Verification items for the finished model (mm, model axes). Coordinates: 2 decimals unless noted, no trailing zeros. Write each loop counter-clockwise with the first axis right and the second up, starting at its lowest first coordinate (ties: lowest second). Pieces come first, ordered by that corner, then holes. Notation, with made-up numbers: (-31.5, 25) -> (-18.5, 25) arc R37 cw to (-18.5, 62) -> close; hole circle Ø3 at (41.25, -6.5). An arc over 180 degrees is marked (long way). Answer in a Markdown table with one row per item.
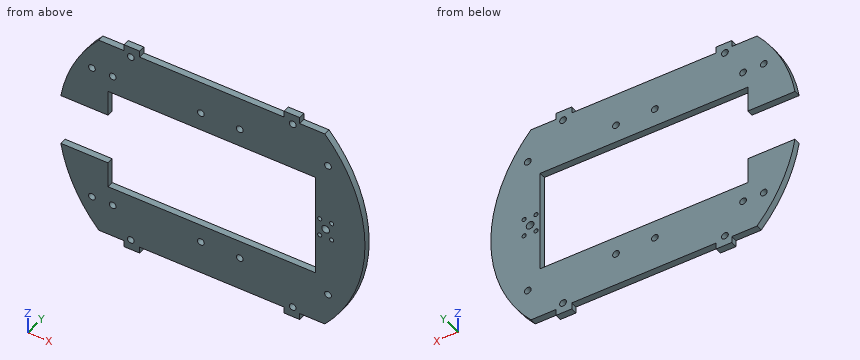
```python
from build123d import *

# Parameters (mm, degrees)
SKETCH1_R           = 1.651
SKETCH1_R_2         = 1.905
SKETCH1_R_3         = 1.016
SKETCH1_W           = 101.6
SKETCH1_H           = 50.8
BOSS_EXTRUDE1_DEPTH = 3.175
SKETCH3_W           = 23.116912814
SKETCH3_H           = 25.4
CUT_EXTRUDE2_DEPTH  = 3.175


with BuildPart() as part:
    # Sketch1 → Boss-Extrude1 (new body)
    with BuildSketch(Plane(origin=(0, 0, 0), x_dir=(1, 0, 0), z_dir=(0, 1, 0))):
        with BuildLine():
            Line((-73.916912814, 12.7), (-73.916912814, -12.7))
            ThreePointArc((-73.916912814, -12.7), (-67.357563081, -32.984218889), (-55.35602635, -50.603461806))
            Line((-55.35602635, -50.603461806), (-42.984152136, -50.603461806))
            Line((-42.984152136, -50.603461806), (-42.984152136, -53.778461806))
            Line((-42.984152136, -53.778461806), (-35.364152136, -53.778461806))
            Line((-35.364152136, -53.778461806), (-35.364152136, -50.603461806))
            Line((-35.364152136, -50.603461806), (35.364152136, -50.603461806))
            Line((35.364152136, -50.603461806), (35.364152136, -53.778461806))
            Line((35.364152136, -53.778461806), (42.984152136, -53.778461806))
            Line((42.984152136, -53.778461806), (42.984152136, -50.603461806))
            Line((42.984152136, -50.603461806), (55.35602635, -50.603461806))
            ThreePointArc((55.35602635, -50.603461806), (75, 0), (55.35602635, 50.603461806))
            Line((55.35602635, 50.603461806), (42.984152136, 50.603461806))
            Line((42.984152136, 50.603461806), (42.984152136, 53.778461806))
            Line((42.984152136, 53.778461806), (35.364152136, 53.778461806))
            Line((35.364152136, 53.778461806), (35.364152136, 50.603461806))
            Line((35.364152136, 50.603461806), (-35.364152136, 50.603461806))
            Line((-35.364152136, 50.603461806), (-35.364152136, 53.778461806))
            Line((-35.364152136, 53.778461806), (-42.984152136, 53.778461806))
            Line((-42.984152136, 53.778461806), (-42.984152136, 50.603461806))
            Line((-42.984152136, 50.603461806), (-55.35602635, 50.603461806))
            ThreePointArc((-55.35602635, 50.603461806), (-67.357563081, 32.984218889), (-73.916912814, 12.7))
        make_face()
        with Locations(Location((13.713087186, 34.29, 0), (0, 0, 270))):
            Circle(SKETCH1_R, mode=Mode.SUBTRACT)
        with Locations(Location((-58.676912814, -34.29, 0), (0, 0, 270))):
            Circle(SKETCH1_R, mode=Mode.SUBTRACT)
        with Locations(Location((-58.676912814, 34.29, 0), (0, 0, 270))):
            Circle(SKETCH1_R, mode=Mode.SUBTRACT)
        with Locations(Location((-39.626912814, 48.698461806, 0), (0, 0, 270))):
            Circle(SKETCH1_R, mode=Mode.SUBTRACT)
        with Locations(Location((39.626912814, 48.698461806, 0), (0, 0, 270))):
            Circle(SKETCH1_R, mode=Mode.SUBTRACT)
        with Locations(Location((-39.626912814, -48.698461806, 0), (0, 0, 270))):
            Circle(SKETCH1_R, mode=Mode.SUBTRACT)
        with Locations(Location((39.626912814, -48.698461806, 0), (0, 0, 270))):
            Circle(SKETCH1_R, mode=Mode.SUBTRACT)
        with Locations(Location((56.893087186, 34.29, 0), (0, 0, 270))):
            Circle(SKETCH1_R, mode=Mode.SUBTRACT)
        with Locations(Location((-48.516912814, 34.29, 0), (0, 0, 270))):
            Circle(SKETCH1_R, mode=Mode.SUBTRACT)
        with Locations(Location((-5.336912814, 34.29, 0), (0, 0, 270))):
            Circle(SKETCH1_R, mode=Mode.SUBTRACT)
        with Locations(Location((-5.336912814, -34.29, 0), (0, 0, 270))):
            Circle(SKETCH1_R, mode=Mode.SUBTRACT)
        with Locations(Location((-48.516912814, -34.29, 0), (0, 0, 270))):
            Circle(SKETCH1_R, mode=Mode.SUBTRACT)
        with Locations(Location((13.713087186, -34.29, 0), (0, 0, 270))):
            Circle(SKETCH1_R, mode=Mode.SUBTRACT)
        with Locations(Location((56.893087186, -34.29, 0), (0, 0, 270))):
            Circle(SKETCH1_R, mode=Mode.SUBTRACT)
        with Locations(Location((55.751543593, 0, 0), (0, 0, 270))):
            Circle(SKETCH1_R_2, mode=Mode.SUBTRACT)
        with Locations(Location((58.671087186, 4.318, 0), (0, 0, 270))):
            Circle(SKETCH1_R_3, mode=Mode.SUBTRACT)
        with Locations(Location((58.671087186, -4.318, 0), (0, 0, 270))):
            Circle(SKETCH1_R_3, mode=Mode.SUBTRACT)
        with Locations(Location((52.832, -4.318, 0), (0, 0, 270))):
            Circle(SKETCH1_R_3, mode=Mode.SUBTRACT)
        with Locations(Location((52.832, 4.318, 0), (0, 0, 270))):
            Circle(SKETCH1_R_3, mode=Mode.SUBTRACT)
        Rectangle(SKETCH1_W, SKETCH1_H, mode=Mode.SUBTRACT)
    extrude(amount=BOSS_EXTRUDE1_DEPTH)

    # Sketch3 → Cut-Extrude2 (cut)
    with BuildSketch(Plane(origin=(0, 3.175, 0), x_dir=(1, 0, 0), z_dir=(0, 1, 0))):
        with Locations((-62.358456407, 0)):
            Rectangle(SKETCH3_W, SKETCH3_H)
    extrude(amount=-CUT_EXTRUDE2_DEPTH, mode=Mode.SUBTRACT)


solid = part.part
```
1. Sectioned sample at C-C, the plane z = -34.29. Record the cut outline in (x, y) (3 decimals), and give its area (3 significant figures).
Findings below:
| item | result |
|---|---|
| outline | (-66.702, 0) -> (-60.328, 0) -> (-60.328, 3.175) -> (-66.702, 3.175) -> close; (-57.026, 0) -> (-50.168, 0) -> (-50.168, 3.175) -> (-57.026, 3.175) -> close; (-46.866, 0) -> (-6.988, 0) -> (-6.988, 3.175) -> (-46.866, 3.175) -> close; (-3.686, 0) -> (12.062, 0) -> (12.062, 3.175) -> (-3.686, 3.175) -> close; (15.364, 0) -> (55.242, 0) -> (55.242, 3.175) -> (15.364, 3.175) -> close; (58.544, 0) -> (66.702, 0) -> (66.702, 3.175) -> (58.544, 3.175) -> close |
| area | 371 mm² |
2. Go/stop test with flat-tipped pins: pin 1 (2.5 mm diameter, centred on x = -5.34, z = 34.29, fed in from -Y); pin 2 (1 mm diameter, centred on x = 51, y = 1, fed in from -Z); pin 3 (1 mm diameter, centred on y = 1, z = 39, fed in from +X); pin 4 (1.6 mm diameter, centred on x = 24.5, y = 1, fed in from +Z). Record where each tip stops, or that it passes through.
Findings below:
| item | result |
|---|---|
| pin 1 | passes through |
| pin 2 | stops at z = -50.6 |
| pin 3 | stops at x = 64.36 |
| pin 4 | stops at z = 50.6 |
3. Sectioned sample at B-B, the plane x = 33.5. Record the cut outline in (y, z) (3 decimals).
Findings below:
| item | result |
|---|---|
| outline | (0, -50.603) -> (3.175, -50.603) -> (3.175, -25.4) -> (0, -25.4) -> close; (0, 25.4) -> (3.175, 25.4) -> (3.175, 50.603) -> (0, 50.603) -> close |
4. Sectioned sample at A-A, the plane z = 0. Record the cut outline in (x, y) (3 decimals).
Findings below:
| item | result |
|---|---|
| outline | (50.8, 0) -> (53.847, 0) -> (53.847, 3.175) -> (50.8, 3.175) -> close; (57.657, 0) -> (75, 0) -> (75, 3.175) -> (57.657, 3.175) -> close |
5. Sectioned sample at D-D, the plane y = 1.2. Count the separate pieces of the cut face and the enclosed holes in it, and give its area (3 significant figures).
Findings below:
| item | result |
|---|---|
| separate pieces | 1 |
| enclosed holes | 19 |
| area | 8,120 mm² |
6. Material ranges on probe 1 along Z at (x, y) = (-25, 1.75); probe 2 along X at (y, z) = (1.85, 4); probe 3 along X at (y, z) = (1.3, 34.29), recorded low to high. Write a range as from..to.
Findings below:
| item | result |
|---|---|
| probe 1 | z = -50.6..-25.4, 25.4..50.6 |
| probe 2 | x = 50.8..51.87, 53.8..57.71, 59.64..74.89 |
| probe 3 | x = -66.7..-60.33, -57.03..-50.17, -46.87..-6.99, -3.69..12.06, 15.36..55.24, 58.54..66.7 |
